Here's the drawing with two shaded views (mm, measured from the low corner). I have some questions. A direction names the side the tool comes from. Coordinates: 2 decimals unless noted, no trailing zeros. Write each loop counter-clockwise with the first axis right and the second up, starting at its lowest first coordinate (ties: lowest second). Pieces come first, ordered by that corner, then holes. Notation, with made-up numbers: (69.25, 50.5) -> (97.25, 50.5) arc R6 cw to (97.25, 56.5) -> close; hole circle Ø8 at (59.25, -17.5). An arc over 180 degrees is marked (long way). Use a Markdown table: item, result. Add a question column.
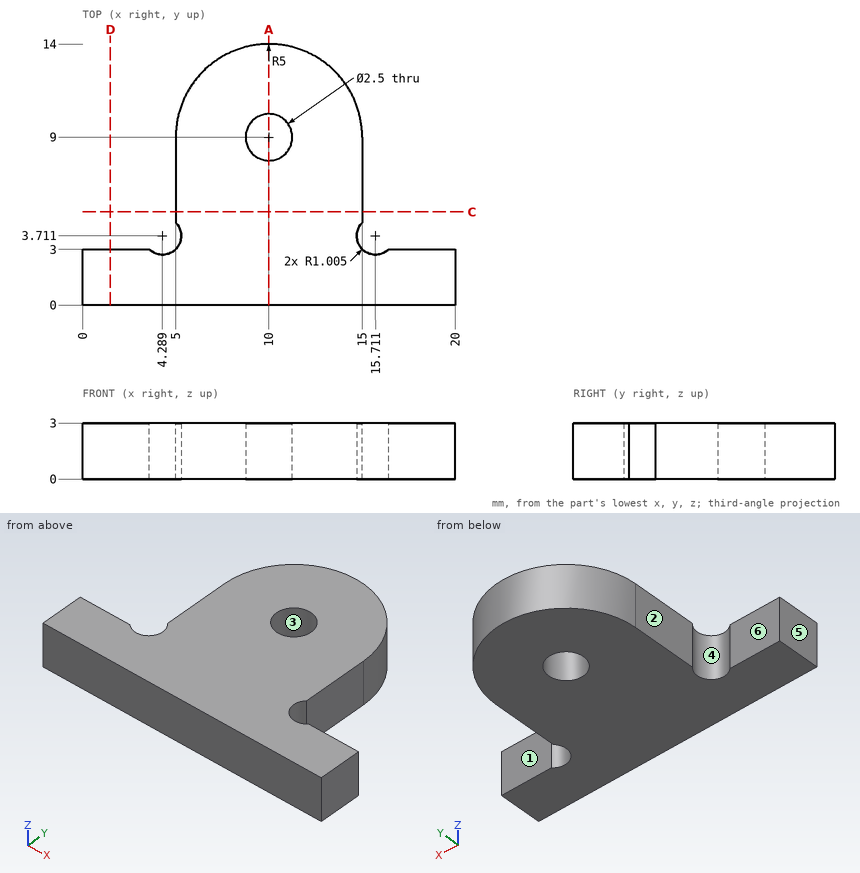
Q1. Suppose I cut it at C-C, the plane y = 5. Write out the boundary of the cut face in (x, z).
Q2. Thinking about a two-plate mould opening in Y: for the marked faces 4, 5 and 6, which applies, released by +Y, released by -Y, zero draft, split by the parting line, or undercut?
Q3. Suppose I cut it at A-A, the plane x = 10. Write out the boundary of the cut face in (y, z), and give its area (3 significant figures).
Q4. Which directions (+Z, -Z, +X, -X, +Y, -Y) give clear straight access to the entire face, cutting with the end or side of a thin tool? Please do the marked faces 1, 2 and 3.
Q5. Will these pins go through, and if not, where does the flat tip stop? pin 1 (0.9 mm diameter, centred on y = 7, z = 1.5, fed in from +X); pin 2 (0.9 mm diameter, centred on x = 2.5, z = 1.5, fed in from +Y).
Q6. Suppose I cut it at D-D, the plane x = 1.5. Write out the boundary of the cut face in (y, z).
Q7. Please list where these lines run through material, in increasing order: line 1 (Y direction, x = 10, z = 0.6); line 2 (X direction, y = 5.5, z = 1.95); line 3 (Y direction, x = 1, z = 0.7).
Answer key:
| question | item | result |
|---|---|---|
| 1 | outline | (5, 0) -> (15, 0) -> (15, 3) -> (5, 3) -> close |
| 2 | face 4 | undercut |
| 2 | face 5 | zero draft |
| 2 | face 6 | released by +Y |
| 3 | outline | (0, 0) -> (7.75, 0) -> (7.75, 3) -> (0, 3) -> close; (10.25, 0) -> (14, 0) -> (14, 3) -> (10.25, 3) -> close |
| 3 | area | 34.5 mm^2 |
| 4 | face 1 | +Z, -Z, +X, +Y |
| 4 | face 2 | +Z, -Z, -X, +Y |
| 4 | face 3 | +Z, -Z |
| 5 | pin 1 | stops at x = 15 |
| 5 | pin 2 | stops at y = 3 |
| 6 | outline | (0, 0) -> (3, 0) -> (3, 3) -> (0, 3) -> close |
| 7 | line 1 | y = 0 to 7.75, 10.25 to 14 |
| 7 | line 2 | x = 5 to 15 |
| 7 | line 3 | y = 0 to 3 |
